Check sheet for the modelled part. Datum: model origin and axes. Units: mm. Coordinates: 2 decimals unless noted, no trailing zeros. Write each loop counter-clockwise with the first axis right and the second up, starting at its lowest first coordinate (ties: lowest second). Pieces come first, ordered by that corner, then holes. Notation, with made-up numbers: (-16, 57) - (-2, 57) arc R17 ccw to (-2, 81) - close; hole circle Ø2 at (39, -21). An arc over 180 degrees is marked (long way). Answer as CSV lines item,"result". Start each with the question number.
from build123d import *

# Parameters (mm, degrees)
BOSS_EXTRUDE1_DEPTH = 16
SKETCH2_R           = 1.35
CUT_EXTRUDE1_DEPTH  = 44.931310019
SKETCH4_R           = 1.742727666
CUT_EXTRUDE3_DEPTH  = 44.931310019
SKETCH3_R           = 3.8
CUT_EXTRUDE2_DEPTH  = 44.931310019
FILLET1_R           = 3
FILLET2_R           = 2
FILLET3_R           = 1.5
CUT_EXTRUDE4_REACH  = 45.662
SKETCH5_R           = 1
CIRPATTERN1_COUNT   = 8
SKETCH6_R           = 1
CUT_EXTRUDE5_DEPTH  = 44.662455396
CIRPATTERN2_COUNT   = 4


with BuildPart() as part:
    # Sketch1 → Boss-Extrude1 (new, symmetric)
    with BuildSketch(Plane.XY):
        Polygon((0, 0), (0, 40), (8.6, 40), (8.6, 38.5), (1.5, 38.5), (1.5, 1.5), (8.6, 1.5), (8.6, 0), align=None)
    extrude(amount=BOSS_EXTRUDE1_DEPTH, both=True)

    # Sketch2 → Cut-Extrude1 (cut, through all)
    with BuildSketch(Plane(origin=(0, 40, 0), x_dir=(1, 0, 0), z_dir=(0, 1, 0))):
        with Locations(Location((6, 11, 0), (0, 0, 180))):
            Circle(SKETCH2_R)
        with Locations(Location((6, -11, 0), (0, 0, 180))):
            Circle(SKETCH2_R)
    extrude(amount=-CUT_EXTRUDE1_DEPTH, mode=Mode.SUBTRACT)

    # Sketch4 → Cut-Extrude3 (cut, through all)
    with BuildSketch(Plane(origin=(0, 40, 0), x_dir=(1, 0, 0), z_dir=(0, 1, 0))):
        with BuildLine():
            Line((8.6, 16), (6, 16))
            ThreePointArc((6, 16), (7.838477631, 15.238477631), (8.6, 13.4))
            Line((8.6, 13.4), (8.6, 16))
        make_face()
        Polygon((0, 18.566066505), (0, 16), (1.742727666, 16), (6, 16), (8.6, 16), (8.6, 13.4), (10.428656455, 13.4), (10.428656455, 18.566066505), align=None)
        with BuildLine():
            ThreePointArc((3.485455332, 14.257272334), (3.476860875, 14.084409002), (3.451162273, 13.91325066))
            ThreePointArc((3.451162273, 13.91325066), (4.352949866, 15.41177182), (6, 16))
            Line((6, 16), (1.742727666, 16))
            ThreePointArc((1.742727666, 16), (2.975022216, 15.489566884), (3.485455332, 14.257272334))
        make_face()
        with Locations((1.742727666, 14.257272334)):
            Circle(SKETCH4_R)
        with BuildLine():
            Line((0, 16), (0, 14.257272334))
            ThreePointArc((0, 14.257272334), (0.510433116, 15.489566884), (1.742727666, 16))
            Line((1.742727666, 16), (0, 16))
        make_face()
        with BuildLine():
            Line((0, 12.514544668), (1.742727666, 12.514544668))
            ThreePointArc((1.742727666, 12.514544668), (0.510433116, 13.024977784), (0, 14.257272334))
            Line((0, 14.257272334), (0, 12.514544668))
        make_face()
    extrude(amount=-CUT_EXTRUDE3_DEPTH, mode=Mode.SUBTRACT)

    # Sketch3 → Cut-Extrude2 (cut, through all)
    with BuildSketch(Plane.ZY):
        with Locations((1.742727666, 20)):
            Circle(SKETCH3_R)
    extrude(amount=-CUT_EXTRUDE2_DEPTH, mode=Mode.SUBTRACT)

    # Fillet1
    fillet1_edges = [part.edges().sort_by_distance(p)[0] for p in [
        (0, 0, 1.742727666),
        (0, 40, 1.742727666),
    ]]
    fillet(fillet1_edges, radius=FILLET1_R)

    # Fillet2
    fillet2_edges = [part.edges().sort_by_distance(p)[0] for p in [
        (8.6, 39.25, 16),
        (8.6, 0.75, 16),
    ]]
    fillet(fillet2_edges, radius=FILLET2_R)

    # Fillet3
    fillet3_edges = [part.edges().sort_by_distance(p)[0] for p in [
        (1.5, 1.5, 1.742727666),
        (1.5, 38.5, 1.742727666),
    ]]
    fillet(fillet3_edges, radius=FILLET3_R)

    # Sketch5 → Cut-Extrude4 (cut, up to next)
    with BuildSketch(Plane(origin=(1.5, 0, 0), x_dir=(0, 0, -1), z_dir=(1, 0, 0)), mode=Mode.PRIVATE) as cut_extrude4_sk1:
        with Locations(Location((-1.742727666, 31, 0), (0, 0, 90))):
            Circle(SKETCH5_R)
    cut_extrude4_tool1 = extrude(cut_extrude4_sk1.sketch, amount=-CUT_EXTRUDE4_REACH, mode=Mode.PRIVATE) & part.part
    cut_extrude4 = cut_extrude4_tool1.solids().sort_by_distance((1.5, 31, 1.742728))[0]
    add(cut_extrude4, mode=Mode.SUBTRACT)

    # CirPattern1: Cut-Extrude4 ×8 about axis
    cirpattern1_axis = Axis((0, 20, 1.742727666), (1, 0, 0))
    for i in range(1, CIRPATTERN1_COUNT):
        add(cut_extrude4.rotate(cirpattern1_axis, i * 360 / CIRPATTERN1_COUNT), mode=Mode.SUBTRACT)

    # Sketch6 → Cut-Extrude5 (cut, through all)
    with BuildSketch(Plane(origin=(1.5, 0, 0), x_dir=(0, 0, -1), z_dir=(1, 0, 0))):
        with Locations(Location((-1.742727666, 28, 0), (0, 0, 90))):
            Circle(SKETCH6_R)
    cut_extrude5 = extrude(amount=-CUT_EXTRUDE5_DEPTH, mode=Mode.SUBTRACT)

    # CirPattern2: Cut-Extrude5 ×4 about axis
    cirpattern2_axis = Axis((0, 20, 1.742727666), (1, 0, 0))
    for i in range(1, CIRPATTERN2_COUNT):
        add(cut_extrude5.rotate(cirpattern2_axis, i * 360 / CIRPATTERN2_COUNT), mode=Mode.SUBTRACT)


solid = part.part
(1) Cross-section at D-D on z = 4.5. Record the boundary of the cut face in (x, y).
(2) Material ranges on probe 1 along Z at (x, y) = (6, 39.7); probe 2 along Y at (x, z) = (8.25, -12.5); probe 3 along Z at (x, y) = (0.85, 31), recorded low to high. Write a range as from..to.
(3) Cross-section at A-A on y = 9. Record the boundary of the cut face in (x, z).
(4) Go/stop test with flat-tipped pins: P1, Ø1.4, axis at x = 1, y = 10.5, coming from the -Z side; P2, Ø2.5, axis at y = 31, z = 1.74, coming from the +X side. Record where each tip stops, or that it passes through.
(5) Cross-section at C-C on z = -4.5. Record the boundary of the cut face in (x, y), plus the area to 3 significant figures.
(6) Cross-section at B-B on y = 20. Record the boundary of the cut face in (x, z), plus the area to 3 significant figures.
(7) Release check for a two-part mould opening along Y. For faces 1 (the face through (0.86, 0.9, 1.68)), 2 (the face through (0.86, 39.1, 1.27)), 3 (the face through (0.76, 13.015, -6.644)), 4 (the face through (0.8, 13, 1.7)) record: pulls with the +Y half, pulls with the -Y half, needs draft (parallel to the pull), parting line crosses it, or undercut.
Checked values:
1,outline,"(0, 3) arc R3 ccw to (3, 0) - (8.6, 0) - (8.6, 1.5) - (3, 1.5) arc R1.5 cw to (1.5, 3) - (1.5, 17.39) - (0, 17.39) - close; (0, 22.61) - (1.5, 22.61) - (1.5, 37) arc R1.5 cw to (3, 38.5) - (8.6, 38.5) - (8.6, 40) - (3, 40) arc R3 ccw to (0, 37) - close"
2,probe 1,"-16..-12.35, -9.65..9.65, 12.35..16"
2,probe 2,"0..1.5, 38.5..40"
2,probe 3,"-12.51..0.74, 2.74..16"
3,outline,"(0, -12.51) - (1.5, -12.51) - (1.5, 0.74) - (0, 0.74) - close; (0, 2.74) - (1.5, 2.74) - (1.5, 16) - (0, 16) - close"
4,P1,"z = -12.51"
4,P2,"x = 1.5"
5,outline,"(0, 3) arc R3 ccw to (3, 0) - (8.6, 0) - (8.6, 1.5) - (3, 1.5) arc R1.5 cw to (1.5, 3) - (1.5, 37) arc R1.5 cw to (3, 38.5) - (8.6, 38.5) - (8.6, 40) - (3, 40) arc R3 ccw to (0, 37) - close"
5,area,"78.4 mm^2"
6,outline,"(0, -12.51) - (1.5, -12.51) - (1.5, -10.26) - (0, -10.26) - close; (0, -8.26) - (1.5, -8.26) - (1.5, -7.26) - (0, -7.26) - close; (0, -5.26) - (1.5, -5.26) - (1.5, -2.06) - (0, -2.06) - close; (0, 5.54) - (1.5, 5.54) - (1.5, 8.74) - (0, 8.74) - close; (0, 10.74) - (1.5, 10.74) - (1.5, 11.74) - (0, 11.74) - close; (0, 13.74) - (1.5, 13.74) - (1.5, 16) - (0, 16) - close"
6,area,"19.4 mm^2"
7,face 1,"pulls with the -Y half"
7,face 2,"pulls with the +Y half"
7,face 3,"undercut"
7,face 4,"undercut"
